Can you work these out from the model? Positions are in its coordinate system, mm. Face numbers are marked on the shaded views. Give positions to 0.01 mm unless a question says otherwise; leave off trailing zeros. Write each loop counter-clockwise with the first axis right and the second up, starting at its lowest first coordinate (ties: lowest second). Pieces come first, ordered by that corner, then holes. Notation, with made-up numbers: (58, -34.5) -> (85, -34.5) arc R9 cw to (85, -20.5) -> close; hole circle Ø8 at (84, 28.25). An arc over 180 degrees is marked (long way). Answer as CSV lines item,"result". Start each with the question number.
1. If we section it at A-A on z = 0: Write out the boundary of the cut face in (x, y), plus the area to 3 significant figures.
2. If we section it at C-C on z = 7: Write out the boundary of the cut face in (x, y), plus the area to 3 significant figures.
3. I need wall thicknesses on line 1 (Z direction, x = 134, y = 0); line 2 (X direction, y = 0, z = 9.6); line 3 (Y direction, x = 159.5, z = -7.5). Which ranges of each line are inside material? Lowest first, please. Write a range as [from, to].
4. I'm going to push flat-ended pins straight in: P1, Ø2, axis at x = 163.5, y = -6.5, coming from the -Z side; P2, Ø10, axis at x = 89, y = 7, coming from the -Z side; P3, Ø1, axis at x = 56, z = 6.5, coming from the -Y side. Where does each tip first touch, or does it pass through?
5. If we section it at B-B on x = 59: Write out the boundary of the cut face in (y, z).
6. If we mould it in two halves opening along Z, with no side actions, what happens to the marked faces 1 and 2? For each: pulls with the +Z half, pulls with the -Z half, needs draft (parallel to the pull), parting line crosses it, or undercut.
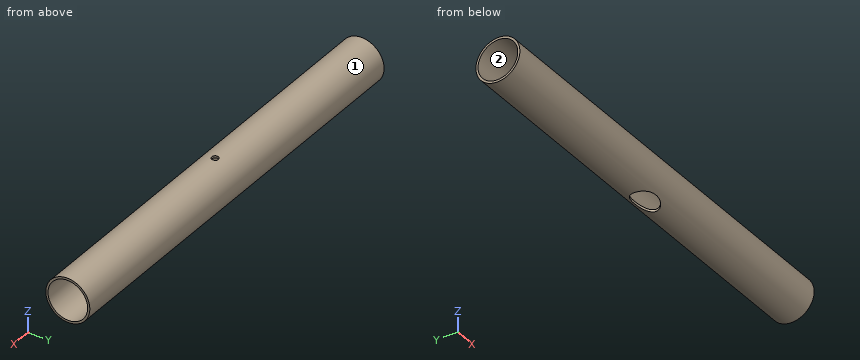
```python
from build123d import *

# Parameters (mm, degrees)
F0_R     = 10.15
F1_DEPTH = 195
F2_R     = 9.15
F3_DEPTH = 195.001
F5_DEPTH = 10.151
F6_R     = 1.55
F7_DEPTH = 10.151


with BuildPart() as f1:
    # F0 (on Right) → F1 (new body)
    with BuildSketch(Plane.YZ):
        Circle(F0_R)
    extrude(amount=F1_DEPTH)

    # F2 (on face) → F3 (cut, through all)
    with BuildSketch(Plane.YZ.offset(195)):
        Circle(F2_R)
    extrude(amount=-F3_DEPTH, mode=Mode.SUBTRACT)

    # F4 (on Top) → F5 (cut, through all)
    with BuildSketch(Plane.XY):
        with BuildLine():
            add(Edge.make_bspline(
                [(105, 0), (105, 8.660254), (93.75, 4.330127), (82.5, 0), (93.75, -4.330127), (105, -8.660254), (105, 0)],
                knots=[0, 0, 0, 2.094395, 2.094395, 4.18879, 4.18879, 6.283185, 6.283185, 6.283185], degree=2, weights=[1, 0.5, 1, 0.5, 1, 0.5, 1]))
        make_face()
    extrude(amount=-F5_DEPTH, mode=Mode.SUBTRACT)

    # F6 (on Top) → F7 (cut, through all)
    with BuildSketch(Plane.XY):
        with Locations((97.5, 0)):
            Circle(F6_R)
    extrude(amount=F7_DEPTH, mode=Mode.SUBTRACT)


solid = f1.part
```
Computed values:
1,outline,"(0, -10.15) -> (195, -10.15) -> (195, -9.15) -> (0, -9.15) -> close; (0, 9.15) -> (195, 9.15) -> (195, 10.15) -> (0, 10.15) -> close"
1,area,"390 mm2"
2,outline,"(0, -7.35) -> (195, -7.35) -> (195, -5.89) -> (0, -5.89) -> close; (0, 5.89) -> (195, 5.89) -> (195, 7.35) -> (0, 7.35) -> close"
2,area,"568 mm2"
3,line 1,"z = [-10.15, -9.15], [9.15, 10.15]"
3,line 2,"x = [0, 95.95], [99.05, 195]"
3,line 3,"y = [-6.84, -5.24], [5.24, 6.84]"
4,P1,"stops at z = -8.53"
4,P2,"stops at z = -9.95"
4,P3,"stops at y = -8.19"
5,outline,"circle Ø20.3 at (0, 0); hole circle Ø18.3 at (0, 0)"
6,face 1,"parting line crosses it"
6,face 2,"undercut"
